Source: CAD feature listing. Evaluate the final solid. Frame: model axes, mm. Face numbers are marked on the shaded views. A direction names the side the tool comes from. Give positions to 0.01 mm unless a question says otherwise; leave off trailing zeros. Loops run counter-clockwise (first coordinate to the right, second up) from the corner with the lowest first, then second, coordinate; pieces in that order, holes last. Notation, with made-up numbers: (5.25, -25) -> (60.25, -25) arc R14 cw to (60.25, -19) -> close; hole circle Ø11 at (-25, -2.75). An arc over 180 degrees is marked (long way). Return JSON: item names as keys, results as strings. Group by question number.
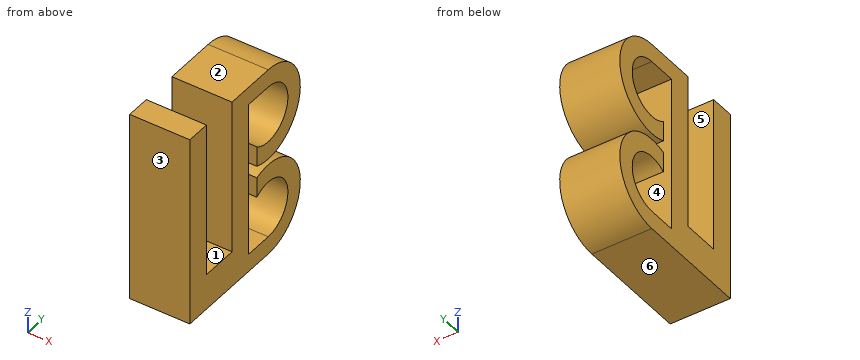
```python
from build123d import *

# Parameters (mm, degrees)
BOSS_EXTRUDE1_DEPTH = 5
BOSS_EXTRUDE2_DEPTH = 5


with BuildPart() as part:
    # Sketch1 → Boss-Extrude1 (new body)
    with BuildSketch(Plane(origin=(0, 0, 0), x_dir=(0, 0, -1), z_dir=(1, 0, 0))):
        with BuildLine():
            Line((-7.997844187, 2.375), (-7.997844187, -2))
            Line((-7.997844187, -2), (7.997844187, -2))
            Line((7.997844187, -2), (7.997844187, 2.375))
            ThreePointArc((7.997844187, 2.375), (3.423879317, 6.186439769), (0.5, 1))
            Line((0.5, 1), (2.186352513, 1))
            ThreePointArc((2.186352513, 1), (3.401228889, 4.637718799), (6.497844187, 2.375))
            Line((6.497844187, 2.375), (6.497844187, 0))
            Line((6.497844187, 0), (-6.497844187, 0))
            Line((-6.497844187, 0), (-6.497844187, 2.375))
            ThreePointArc((-6.497844187, 2.375), (-3.401228889, 4.637718799), (-2.186352513, 1))
            Line((-2.186352513, 1), (-0.5, 1))
            ThreePointArc((-0.5, 1), (-3.423879317, 6.186439769), (-7.997844187, 2.375))
        make_face()
    extrude(amount=BOSS_EXTRUDE1_DEPTH)

    # Sketch2 → Boss-Extrude2 (add)
    with BuildSketch(Plane.ZY):
        Polygon((-7.997844187, -2), (-7.997844187, -7.1), (7.997844187, -7.1), (7.997844187, -5.1), (-4.997844187, -5.1), (-4.997844187, -2), align=None)
    extrude(amount=-BOSS_EXTRUDE2_DEPTH)


solid = part.part
```
1) Cut plane A-A on y = 0.5. Return loops of the section in (x, z).
2) Cut plane B-B on z = 2.75. Return loops of the section in (x, y).
3) Mould query, pull axis Y, two halves, no side actions, for the marked faces 1, 2 and 3. Classes: released by +Y, released by -Y, zero draft, split by the parting line, or undercut.
4) Material intervals for line 1 (Z direction, x = 4.5, y = 0.75); line 2 (Z direction, x = 2.3, y = 4); line 3 (Y direction, x = 1.1, z = 1.25), sorted ascending.
5) Cut plane D-D on y = 2. Return loops of the section in (x, z), then the cut area to 3 significant figures.
6) Reachability of the marked faces 4, 5 and 6 from +Z, -Z, +X, -X, +Y, -Y: full face, straight path, thin tool, end or side. Return the list, or none.
7) Cut plane C-C on x = 0.7. Return loops of the section in (y, z) (3 decimals).
8) Contact query for flat-ended pins moving along their axis: P1, Ø0.9, axis at x = 3, y = -4, coming from the +Z side; P2, Ø1, axis at x = 3.5, z = 1, coming from the +Y side; P3, Ø1, axis at x = 4.5, z = -6, coming from the +Y side. Output: stop coordinate, or through.
Calculated:
{
 "1": {"outline": "(0, -8) -> (5, -8) -> (5, -6.5) -> (0, -6.5) -> close; (0, 6.5) -> (5, 6.5) -> (5, 8) -> (0, 8) -> close"},
 "2": {"outline": "(0, -7.1) -> (5, -7.1) -> (5, -5.1) -> (0, -5.1) -> close; (0, -2) -> (5, -2) -> (5, 0) -> (0, 0) -> close; (0, 4.31) -> (5, 4.31) -> (5, 6) -> (0, 6) -> close"},
 "3": {"face 1": "undercut", "face 2": "zero draft", "face 3": "released by -Y"},
 "4": {"line 1": "-8 to -6.5, 6.5 to 8", "line 2": "-7.64 to -5.85, -2.39 to -0.61, 0.61 to 2.39, 5.85 to 7.64", "line 3": "-7.1 to -5.1, -2 to 0, 1 to 4.98"},
 "5": {"outline": "(0, -8) -> (5, -8) -> (5, -6.5) -> (0, -6.5) -> close; (0, -1.78) -> (5, -1.78) -> (5, -0.27) -> (0, -0.27) -> close; (0, 0.27) -> (5, 0.27) -> (5, 1.78) -> (0, 1.78) -> close; (0, 6.5) -> (5, 6.5) -> (5, 8) -> (0, 8) -> close", "area": "30.1 mm2"},
 "6": {"face 4": "+X, -X", "face 5": "+Z, +X, -X", "face 6": "-Z, +X, -X, +Y, -Y"},
 "7": {"outline": "(-7.1, -7.998) -> (2.375, -7.998) arc R3.875 ccw (long way) to (1, -0.5) -> (1, -2.186) arc R2.375 cw (long way) to (2.375, -6.498) -> (0, -6.498) -> (0, 6.498) -> (2.375, 6.498) arc R2.375 cw (long way) to (1, 2.186) -> (1, 0.5) arc R3.875 ccw (long way) to (2.375, 7.998) -> (-2, 7.998) -> (-2, -4.998) -> (-5.1, -4.998) -> (-5.1, 7.998) -> (-7.1, 7.998) -> close"},
 "8": {"P1": "z = -5", "P2": "y = 5.23", "P3": "y = 6"}
}
